```python
from build123d import *

# Parameters (mm, degrees)
SKETCH1_W                       = 10.823103443
SKETCH1_H                       = 51.052518719
BOSS_EXTRUDE1_DEPTH             = 50.8
SKETCH2_W                       = 177.8
SKETCH2_H                       = 31.75
BOSS_EXTRUDE2_DEPTH             = 7.62
F_1_2_START                     = -59.944
F_1_2_CLEARANCE_HOLE1_OUTLINE_R = 6.74624
F_1_2_CLEARANCE_HOLE1_DEPTH     = 7.62
SKETCH8_R                       = 4.4323
CUT_EXTRUDE2_DEPTH              = 138.353334223
SKETCH9_R                       = 4.4323
CUT_EXTRUDE3_DEPTH              = 132.62094122


# Read off the part's stored shape, not the designer's step: 1/2 Clearance Hole1
with BuildPart() as part:
    # Sketch1 → Boss-Extrude1 (new, symmetric)
    with BuildSketch(Plane.XY):
        with Locations((-64.692448278, -34.41774064)):
            Rectangle(SKETCH1_W, SKETCH1_H)
        with BuildLine():
            ThreePointArc((-2e-09, -59.944), (-39.117081832, -45.421768404), (-59.280896557, -8.891481281))
            Line((-59.280896557, -8.891481281), (-59.280896557, -59.944))
            Line((-59.280896557, -59.944), (-2e-09, -59.944))
        make_face()
        with BuildLine():
            Line((-50.42609614, -8.891481281), (-59.280896557, -8.891481281))
            ThreePointArc((-59.280896557, -8.891481281), (-39.117081832, -45.421768404), (-2e-09, -59.944))
            ThreePointArc((-2e-09, -59.944), (42.386808891, -42.386808892), (59.944, 0))
            ThreePointArc((59.944, 0), (59.902397652, 2.232911009), (59.777648353, 4.462722648))
            Line((59.777648353, 4.462722648), (51.009153275, 4.462722648))
            ThreePointArc((51.009153275, 4.462722648), (51.155265092, 2.233487109), (51.203999954, 0))
            ThreePointArc((51.203999954, 0), (4.462722648, -51.009153275), (-50.42609614, -8.891481281))
        make_face()
        with BuildLine():
            ThreePointArc((59.944, 0), (42.386808891, -42.386808892), (-2e-09, -59.944))
            Line((-2e-09, -59.944), (59.944, -59.944))
            Line((59.944, -59.944), (59.944, 0))
        make_face()
        with BuildLine():
            Line((70.104, 4.462722648), (59.777648353, 4.462722648))
            ThreePointArc((59.777648353, 4.462722648), (59.902397652, 2.232911009), (59.944, 0))
            Line((59.944, 0), (59.944, -59.944))
            Line((59.944, -59.944), (70.104, -59.944))
            Line((70.104, -59.944), (70.104, 4.462722648))
        make_face()
    extrude(amount=BOSS_EXTRUDE1_DEPTH, both=True)

    # Sketch2 → Boss-Extrude2 (add)
    with BuildSketch(Plane.XZ.offset(59.944)):
        with Locations((0, 66.675)):
            Rectangle(SKETCH2_W, SKETCH2_H)
    boss_extrude2 = extrude(amount=-BOSS_EXTRUDE2_DEPTH)

    # 1/2 Clearance Hole1 outline → 1/2 Clearance Hole1 (cut)
    with BuildSketch(Plane(origin=(0, 0, 0), x_dir=(1, 0, 0), z_dir=(0, 1, 0)).offset(F_1_2_START)):
        with Locations((63.5, -69.85)):
            Circle(F_1_2_CLEARANCE_HOLE1_OUTLINE_R)
        with Locations((-63.5, -69.85)):
            Circle(F_1_2_CLEARANCE_HOLE1_OUTLINE_R)
    f_1_2_clearance_hole1 = extrude(amount=F_1_2_CLEARANCE_HOLE1_DEPTH, mode=Mode.SUBTRACT)

    # Mirror1: Boss-Extrude2, 1/2 Clearance Hole1 across plane
    add(boss_extrude2.mirror(Plane.XY))
    add(f_1_2_clearance_hole1.mirror(Plane.XY), mode=Mode.SUBTRACT)

    # Sketch8 → Cut-Extrude2 (cut, through all)
    with BuildSketch(Plane(origin=(0, 4.462722648, 0), x_dir=(1, 0, 0), z_dir=(0, 1, 0))):
        with Locations(Location((62.484, 31.75, 0), (0, 0, 180))):
            Circle(SKETCH8_R)
        with Locations(Location((62.484, -31.75, 0), (0, 0, 180))):
            Circle(SKETCH8_R)
    extrude(amount=-CUT_EXTRUDE2_DEPTH, mode=Mode.SUBTRACT)

    # Sketch9 → Cut-Extrude3 (cut, through all)
    with BuildSketch(Plane(origin=(0, -8.891481281, 0), x_dir=(1, 0, 0), z_dir=(0, 1, 0))):
        with Locations(Location((-62.484, 31.75, 0), (0, 0, 270))):
            Circle(SKETCH9_R)
        with Locations(Location((-62.484, -31.75, 0), (0, 0, 270))):
            Circle(SKETCH9_R)
    extrude(amount=-CUT_EXTRUDE3_DEPTH, mode=Mode.SUBTRACT)


solid = part.part
```
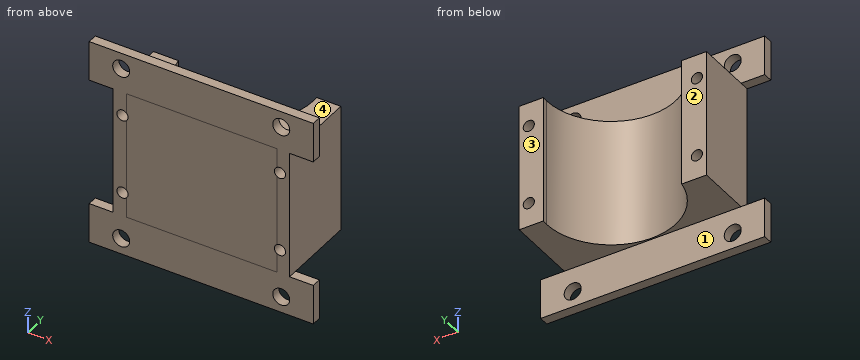
Geometry: final body of the model. Coordinates: model frame, mm. Face numbers are marked on the shaded views. A direction names the side the tool comes from. Round coordinates to 2 decimals unless told otherwise and drop trailing zeros. Loops run counter-clockwise (first coordinate to the right, second up) from the corner with the lowest first, then second, coordinate; pieces in that order, holes last. Notation, with made-up numbers: (1, 42) -> (24, 42) arc R20 ccw to (24, 58) -> close; hole circle Ø3 at (54.25, -19.75). An arc over 180 degrees is marked (long way). Use one line per item in the form item = value. Start each with the question number.
1) First-contact query: P1, Ø3, axis at x = -65.5, z = -52.5, coming from the +Y side; P2, Ø4, axis at y = -41.5, z = 8, coming from the +X side; P3, Ø4, axis at x = -40.5, z = -33, coming from the +Y side; P4, Ø8, axis at x = 62.484, z = -31.75, coming from the +Y side. Flat tips, straight axial feed; report the tip coordinate or a pass-through.
2) Access query for the marked faces 1, 2, 3 and 4. Directions: +Z, -Z, +X, -X, +Y, -Y. A direction counts if a zero-diameter tool reaches every point of the face in a straight line with its end or side. Return the directions, or none.
3) Section C-C on x = 63.5. Output: boundary loops of the cut face in (y, z).
4) Section A-A on z = 69.85. Output: boundary loops of the cut face in (x, y).
5) Section B-B on y = -44. Output: boundary loops of the cut face in (x, z).
6) Line query: L1, parallel to Z at x = -63, y = -53; L2, parallel to X at y = -41, z = 31.75; L3, parallel to Z at x = 39, y = -49. Output: solid intervals per line, ascending.
Response:
q1.P1 = -52.32
q1.P2 = 70.1
q1.P3 = -28.56
q1.P4 = through
q2.face_1 = -Z, +X, -X, +Y
q2.face_2 = +Z, -Z, -X, +Y
q2.face_3 = +Z, -Z, +X, -X, +Y
q2.face_4 = +Z, +X, -X, +Y
q3.outline = (-59.94, -82.55) -> (-52.32, -82.55) -> (-52.32, -76.6) -> (-59.94, -76.6) -> close; (-59.94, -63.1) -> (-52.32, -63.1) -> (-52.32, -50.8) -> (4.46, -50.8) -> (4.46, -36.06) -> (-59.94, -36.06) -> close; (-59.94, -27.44) -> (4.46, -27.44) -> (4.46, 27.44) -> (-59.94, 27.44) -> close; (-59.94, 36.06) -> (4.46, 36.06) -> (4.46, 50.8) -> (-52.32, 50.8) -> (-52.32, 63.1) -> (-59.94, 63.1) -> close; (-59.94, 76.6) -> (-52.32, 76.6) -> (-52.32, 82.55) -> (-59.94, 82.55) -> close
q4.outline = (-88.9, -59.94) -> (-70.25, -59.94) -> (-70.25, -52.32) -> (-88.9, -52.32) -> close; (-56.75, -59.94) -> (56.75, -59.94) -> (56.75, -52.32) -> (-56.75, -52.32) -> close; (70.25, -59.94) -> (88.9, -59.94) -> (88.9, -52.32) -> (70.25, -52.32) -> close
q5.outline = (-70.1, -50.8) -> (-26.19, -50.8) -> (-26.19, 50.8) -> (-70.1, 50.8) -> close; (26.19, -50.8) -> (70.1, -50.8) -> (70.1, 50.8) -> (26.19, 50.8) -> close; hole circle Ø8.86 at (-62.48, -31.75); hole circle Ø8.86 at (-62.48, 31.75); hole circle Ø8.86 at (62.48, -31.75); hole circle Ø8.86 at (62.48, 31.75)
q6.L1 = -82.55 to -76.58, -63.12 to -36.15, -27.35 to 27.35, 36.15 to 63.12, 76.58 to 82.55
q6.L2 = -70.1 to -66.92, -58.05 to -30.67, 30.67 to 58.05, 66.92 to 70.1
q6.L3 = -50.8 to 50.8
